Here's how the part is built. I have some questions about the finished solid (model axes, mm). Face numbers are marked on the shaded views. A direction names the side the tool comes from. Round coordinates to 2 decimals unless told otherwise and drop trailing zeros. Order: outer loops, then holes, each group sorted by start corner. A loop starts at its lowest first (then second) coordinate and runs counter-clockwise, first axis right, second up.
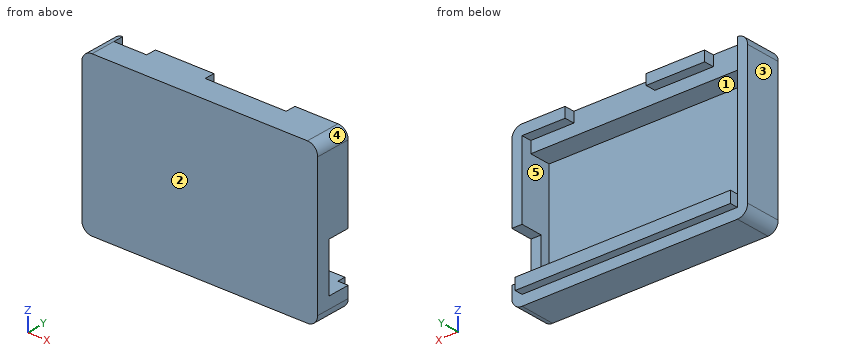
```python
from build123d import *

# Parameters (mm, degrees)
SKETCH1_W            = 57.5
SKETCH1_H            = 38.5
SKETCH1_W_2          = 52.5
SKETCH1_H_2          = 33.5
BOSS_EXTRUDE1_DEPTH  = 10.25
SKETCH10_W           = 52.5
SKETCH10_H           = 33.5
BOSS_EXTRUDE8_DEPTH  = 2.5
SKETCH11_W           = 52.5
SKETCH11_H           = 2.8
BOSS_EXTRUDE9_DEPTH  = 9.75
SKETCH12_W           = 52.5
SKETCH12_H           = 2.8
BOSS_EXTRUDE10_DEPTH = 5.25
SKETCH13_W           = 12
SKETCH13_H           = 5.5
CUT_EXTRUDE1_DEPTH   = 2.5
SKETCH14_W           = 8
SKETCH14_H           = 2.5
SKETCH14_W_2         = 19.75
CUT_EXTRUDE2_DEPTH   = 2.5
SKETCH15_W           = 38.5
SKETCH15_H           = 1.5
CUT_EXTRUDE3_DEPTH   = 57.5
FILLET1_R            = 2.5


with BuildPart() as part:
    # Sketch1 → Boss-Extrude1 (new body)
    with BuildSketch(Plane(origin=(0, 0, 0), x_dir=(1, 0, 0), z_dir=(0, 1, 0))):
        with Locations((28.75, 19.25)):
            Rectangle(SKETCH1_W, SKETCH1_H)
        with Locations((28.75, 19.25)):
            Rectangle(SKETCH1_W_2, SKETCH1_H_2, mode=Mode.SUBTRACT)
    extrude(amount=BOSS_EXTRUDE1_DEPTH)

    # Sketch10 → Boss-Extrude8 (add)
    with BuildSketch(Plane(origin=(0, 0, 0), x_dir=(1, 0, 0), z_dir=(0, 1, 0))):
        with Locations((28.75, 19.25)):
            Rectangle(SKETCH10_W, SKETCH10_H)
    extrude(amount=BOSS_EXTRUDE8_DEPTH)

    # Sketch11 → Boss-Extrude9 (add)
    with BuildSketch(Plane(origin=(0, 2.5, 0), x_dir=(1, 0, 0), z_dir=(0, 1, 0))):
        with Locations((28.75, 34.6)):
            Rectangle(SKETCH11_W, SKETCH11_H)
    extrude(amount=BOSS_EXTRUDE9_DEPTH)

    # Sketch12 → Boss-Extrude10 (add)
    with BuildSketch(Plane(origin=(0, 2.5, 0), x_dir=(1, 0, 0), z_dir=(0, 1, 0))):
        with Locations((28.75, 3.9)):
            Rectangle(SKETCH12_W, SKETCH12_H)
    extrude(amount=BOSS_EXTRUDE10_DEPTH)

    # Sketch13 → Cut-Extrude1 (cut)
    with BuildSketch(Plane(origin=(57.5, 0, 0), x_dir=(0, 0, -1), z_dir=(1, 0, 0))):
        with Locations((27.2, 7.5)):
            Rectangle(SKETCH13_W, SKETCH13_H)
    extrude(amount=-CUT_EXTRUDE1_DEPTH, mode=Mode.SUBTRACT)

    # Sketch14 → Cut-Extrude2 (cut)
    with BuildSketch(Plane(origin=(0, 0, -2.5), x_dir=(-1, 0, 0), z_dir=(0, 0, -1))):
        with Locations((-6.5, 9)):
            Rectangle(SKETCH14_W, SKETCH14_H)
        with Locations((-34.625, 9)):
            Rectangle(SKETCH14_W_2, SKETCH14_H)
    extrude(amount=-CUT_EXTRUDE2_DEPTH, mode=Mode.SUBTRACT)

    # Sketch15 → Cut-Extrude3 (cut)
    with BuildSketch(Plane.ZY):
        with Locations((-19.25, 0.75)):
            Rectangle(SKETCH15_W, SKETCH15_H)
    extrude(amount=-CUT_EXTRUDE3_DEPTH, mode=Mode.SUBTRACT)

    # Fillet1
    fillet1_edges = [part.edges().sort_by_distance(p)[0] for p in [
        (0, 5.875, 0),
        (0, 5.875, -38.5),
        (57.5, 5.875, -38.5),
        (57.5, 5.875, 0),
    ]]
    fillet(fillet1_edges, radius=FILLET1_R)


solid = part.part
```
1. If we section it at A-A, the plane y = 4: Write out the boundary of the cut face in (x, z).
Evaluation:
outline: (0, -36) arc R2.5 ccw to (2.5, -38.5) - (55, -38.5) arc R2.5 ccw to (57.5, -36) - (57.5, -2.5) arc R2.5 ccw to (55, 0) - (2.5, 0) arc R2.5 ccw to (0, -2.5) - close; hole (2.5, -33.2) - (55, -33.2) - (55, -5.3) - (2.5, -5.3) - close
2. If we section it at C-C, the plane y = 6.5: Write out the boundary of the cut face in (x, z).
Evaluation:
outline: (0, -36) arc R2.5 ccw to (2.5, -38.5) - (55, -38.5) arc R2.5 ccw to (57.5, -36) - (57.5, -33.2) - (2.5, -33.2) - (2.5, -5.3) - (55, -5.3) - (55, -21.2) - (57.5, -21.2) - (57.5, -2.5) arc R2.5 ccw to (55, 0) - (2.5, 0) arc R2.5 ccw to (0, -2.5) - close
3. I need wall thicknesses on probe 1 along X at (y, z) = (9, -13.5); probe 2 along Z at (x, y) = (53.5, 5); probe 3 along Z at (x, y) = (21, 8.25). Which ranges of each line are inside material? Lowest first, please.
Evaluation:
probe 1: x = 0 to 2.5, 55 to 57.5
probe 2: z = -38.5 to -33.2, -5.3 to 0
probe 3: z = -38.5 to -33.2, -2.5 to 0
4. On a 3-axis mill with a long thin cutter (end or side, diameter ignored), from which of +Z, -Z, +X, -X, +Y, -Y can I reach the whole of each face in a straight line? I mean the marked faces 1 and 2. Say none if no direction works.
Evaluation:
face 1: +Y
face 2: +Z, -Z, +X, -X, -Y
5. If we mould it in two halves opening along X, with no side actions, what happens to the marked faces 3, 4 and 5? For each: released by +X, released by -X, zero draft, split by the parting line, or undercut.
Evaluation:
face 3: released by -X
face 4: released by +X
face 5: undercut
6. I'm going to push flat-ended pins straight in: P1, Ø6, axis at x = 20.5, z = -18, coming from the +Y side; P2, Ø1.6, axis at x = 23.5, y = 11.5, coming from the -Z side; P3, Ø4, axis at y = 8, z = -24, coming from the +X side. Where does each tip first touch, or does it pass through?
Evaluation:
P1: stops at y = 2.5
P2: stops at z = -36
P3: stops at x = 2.5
7. If we section it at D-D, the plane x = 4.5: Write out the boundary of the cut face in (y, z), and give its area (3 significant figures).
Evaluation:
outline: (1.5, -38.5) - (10.25, -38.5) - (10.25, -36) - (12.25, -36) - (12.25, -33.2) - (2.5, -33.2) - (2.5, -5.3) - (7.75, -5.3) - (7.75, 0) - (1.5, 0) - close
area: 113 mm2
8. If we section it at B-B, the plane z = -6.5: Write out the boundary of the cut face in (x, y).
Evaluation:
outline: (0, 1.5) - (57.5, 1.5) - (57.5, 10.25) - (55, 10.25) - (55, 2.5) - (2.5, 2.5) - (2.5, 10.25) - (0, 10.25) - close
